Verification items for the finished model (mm, model axes). Face numbers are marked on the shaded views. A direction names the side the tool comes from. Give positions to 0.01 mm unless a question says otherwise; leave off trailing zeros. Order: outer loops, then holes, each group sorted by start corner. A loop starts at its lowest first (then second) coordinate and runs counter-clockwise, first axis right, second up.
from build123d import *

# Parameters (mm, degrees)
F0_R     = 3.175
F1_DEPTH = 6.35


# Not quite as in the source:
# - the program builds the solid bodies; features that only make, move or delete a surface that nothing else refers to are left out


with BuildPart() as f1:
    # F0 (on Front) → F1 (new body)
    with BuildSketch(Plane.XZ):
        with BuildLine():
            ThreePointArc((4.4289185951, -8.4326926351), (8.1520265768, -4.9264680747), (9.525, 0))
            ThreePointArc((9.525, 0), (6.936415596, 6.5277686601), (0.5776480463, 9.5074679981))
            ThreePointArc((0.5776480463, 9.5074679981), (-9.3128281564, -1.9992140281), (4.4289185951, -8.4326926351))
        make_face()
        Circle(F0_R, mode=Mode.SUBTRACT)
        with BuildLine():
            ThreePointArc((0.5776480463, 9.5074679981), (6.936415596, 6.5277686601), (9.525, 0))
            ThreePointArc((9.525, 0), (8.1520265768, -4.9264680747), (4.4289185951, -8.4326926351))
            Line((4.4289185951, -8.4326926351), (20.4848255962, 0))
            Line((20.4848255962, 0), (31.5823644939, 5.8285174748))
            Line((31.5823644939, 5.8285174748), (35.56, 0))
            Line((35.56, 0), (31.5823644939, 7.623705267))
            Line((31.5823644939, 7.623705267), (30.6727180917, 7.6789729226))
            Line((30.6727180917, 7.6789729226), (0.5776480463, 9.5074679981))
        make_face()
    extrude(amount=F1_DEPTH)


solid = f1.part
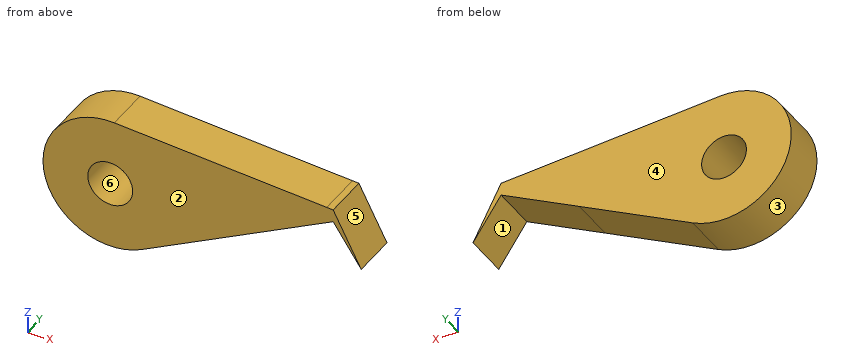
(1) Section check C-C, the plane z = 4. Enter the section's corners in (x, y), then the cut area to 3 significant figures.
Solved:
outline: (-8.64, -6.35) - (28.1, -6.35) - (28.1, 0) - (-8.64, 0) - close; (32.83, -6.35) - (33.47, -6.35) - (33.47, 0) - (32.83, 0) - close
area: 237 mm2
(2) Section check D-D, the plane x = 27.5. Enter the section's corners in (y, z), then the cut area to 3 significant figures.
Solved:
outline: (-6.35, 3.68) - (0, 3.68) - (0, 7.87) - (-6.35, 7.87) - close
area: 26.6 mm2
(3) Section check B-B, the plane y = -3. Enter the section's corners in (x, z) (3 decimals), then the cut area to 3 significant figures.
Solved:
outline: (0.578, 9.507) arc R9.525 ccw (long way) to (4.429, -8.433) - (31.582, 5.829) - (35.56, 0) - (31.582, 7.624) - close; hole circle Ø6.35 at (0, 0)
area: 461 mm2
(4) Section check A-A, the plane x = 0. Enter the section's corners in (y, z) (3 decimals), then the cut area to 3 significant figures.
Solved:
outline: (-6.35, -9.525) - (0, -9.525) - (0, -3.175) - (-6.35, -3.175) - close; (-6.35, 3.175) - (0, 3.175) - (0, 9.525) - (-6.35, 9.525) - close
area: 80.6 mm2
(5) Release check for a two-part mould opening along Z. For the marked faces 3, 4, 5 and 6 record: pulls with the +Z half, pulls with the -Z half, needs draft (parallel to the pull), parting line crosses it, or undercut.
Solved:
face 3: parting line crosses it
face 4: needs draft
face 5: pulls with the +Z half
face 6: undercut
(6) Set-up check for the marked faces 1 and 2: record each of +Z, -Z, +X, -X, +Y, -Y from which the full face is reachable in a straight line by a thin tool's end or side.
Solved:
face 1: -Z, +Y, -Y
face 2: +Z, -Z, +X, -X, -Y
(7) Scan lines: line 1 (Z direction, x = 0, y = -4) (3 decimals); line 2 (X direction, y = -1.25, z = 2.5); line 3 (Z direction, x = 2, y = -0.5). Record each from-to range of solid material in increasing order.
Solved:
line 1: z = -9.525 to -3.175, 3.175 to 9.525
line 2: x = -9.19 to -1.96, 1.96 to 25.24, 33.85 to 34.26
line 3: z = -9.31 to -2.47, 2.47 to 9.42
(8) Go/stop test with flat-tipped pins: pin 1 (3 mm diameter, centred on y = -1, z = -2, fed in from +X); pin 2 (1.5 mm diameter, centred on x = -3, y = -4, fed in from -Z); pin 3 (3 mm diameter, centred on x = 5.5, y = -1, fed in from +Z). Record where each tip stops, or that it passes through.
Solved:
pin 1: stops at x = 19.53
pin 2: stops at z = -9.26
pin 3: stops at z = 9.3
